from build123d import *

# Parameters (mm, degrees)
BOSS_EXTRUDE1_DEPTH = 124.46
BOSS_EXTRUDE2_START = 127
BOSS_EXTRUDE2_DEPTH = 2.54
BOSS_EXTRUDE3_START = -124.46
BOSS_EXTRUDE3_DEPTH = 2.54
CUT_EXTRUDE1_START  = 19.05
SKETCH4_R           = 6.35
CUT_EXTRUDE1_DEPTH  = 2.54
FILLET1_R           = 2.54
FILLET2_R           = 2.54


with BuildPart() as part:
    # Sketch1 → Boss-Extrude1 (new, symmetric)
    with BuildSketch(Plane(origin=(0, 0, 0), x_dir=(0, 0, -1), z_dir=(1, 0, 0))):
        with BuildLine():
            Line((-16.51, 38.1), (-19.05, 38.1))
            Line((-19.05, 38.1), (-19.05, 2.54))
            ThreePointArc((-19.05, 2.54), (-18.306051224, 0.743948776), (-16.51, 0))
            Line((-16.51, 0), (0, 0))
            Line((0, 0), (0, 1.016))
            Line((0, 1.016), (-6.35, 1.016))
            Line((-6.35, 1.016), (-6.35, 2.54))
            Line((-6.35, 2.54), (-16.51, 2.54))
            Line((-16.51, 2.54), (-16.51, 38.1))
        make_face()
        with BuildLine():
            Line((0, 1.016), (0, 0))
            Line((0, 0), (16.51, 0))
            ThreePointArc((16.51, 0), (18.306051224, 0.743948776), (19.05, 2.54))
            Line((19.05, 2.54), (19.05, 38.1))
            Line((19.05, 38.1), (16.51, 38.1))
            Line((16.51, 38.1), (16.51, 2.54))
            Line((16.51, 2.54), (6.35, 2.54))
            Line((6.35, 2.54), (6.35, 1.016))
            Line((6.35, 1.016), (0, 1.016))
        make_face()
    extrude(amount=BOSS_EXTRUDE1_DEPTH, both=True)

    # Sketch3 → Boss-Extrude2 (add)
    with BuildSketch(Plane(origin=(0, 0, 0), x_dir=(0, 0, -1), z_dir=(1, 0, 0)).offset(BOSS_EXTRUDE2_START)):
        with BuildLine():
            Line((0, 38.1), (-19.05, 38.1))
            Line((-19.05, 38.1), (-19.05, 2.54))
            ThreePointArc((-19.05, 2.54), (-18.306051224, 0.743948776), (-16.51, 0))
            Line((-16.51, 0), (0, 0))
            Line((0, 0), (0, 38.1))
        make_face()
        with BuildLine():
            Line((19.05, 38.1), (0, 38.1))
            Line((0, 38.1), (0, 0))
            Line((0, 0), (16.51, 0))
            ThreePointArc((16.51, 0), (18.306051224, 0.743948776), (19.05, 2.54))
            Line((19.05, 2.54), (19.05, 38.1))
        make_face()
    extrude(amount=-BOSS_EXTRUDE2_DEPTH)

    # Sketch3<4> → Boss-Extrude3 (add)
    with BuildSketch(Plane(origin=(0, 0, 0), x_dir=(0, 0, -1), z_dir=(1, 0, 0)).offset(BOSS_EXTRUDE3_START)):
        with BuildLine():
            Line((0, 38.1), (-19.05, 38.1))
            Line((-19.05, 38.1), (-19.05, 2.54))
            ThreePointArc((-19.05, 2.54), (-18.306051224, 0.743948776), (-16.51, 0))
            Line((-16.51, 0), (0, 0))
            Line((0, 0), (0, 38.1))
        make_face()
        with BuildLine():
            Line((19.05, 38.1), (0, 38.1))
            Line((0, 38.1), (0, 0))
            Line((0, 0), (16.51, 0))
            ThreePointArc((16.51, 0), (18.306051224, 0.743948776), (19.05, 2.54))
            Line((19.05, 2.54), (19.05, 38.1))
        make_face()
    extrude(amount=-BOSS_EXTRUDE3_DEPTH)

    # Sketch4 → Cut-Extrude1 (cut)
    with BuildSketch(Plane.XY.offset(CUT_EXTRUDE1_START)):
        with Locations((-116.84, 10.16)):
            Circle(SKETCH4_R)
    extrude(amount=-CUT_EXTRUDE1_DEPTH, mode=Mode.SUBTRACT)

    # Fillet1
    fillet1_edges = [part.edges().sort_by_distance(p)[0] for p in [
        (-127, 0.743948776, -18.306051224),
        (-127, 0, 0),
        (-127, 0.743948776, 18.306051224),
        (-127, 20.32, 19.05),
        (-127, 20.32, -19.05),
    ]]
    fillet(fillet1_edges, radius=FILLET1_R)

    # Fillet2
    fillet2_edges = [part.edges().sort_by_distance(p)[0] for p in [
        (127, 0, 0),
        (127, 20.32, 19.05),
        (127, 0.743948776, -18.306051224),
        (127, 20.32, -19.05),
        (127, 0.743948776, 18.306051224),
    ]]
    fillet(fillet2_edges, radius=FILLET2_R)


solid = part.part
Verification items for the finished model (mm, model axes). A direction names the side the tool comes from. Round coordinates to 2 decimals unless told otherwise and drop trailing zeros. Order: outer loops, then holes, each group sorted by start corner. A loop starts at its lowest first (then second) coordinate and runs counter-clockwise, first axis right, second up. Notation, with made-up numbers: (36, -25) -> (67, -25) arc R22 cw to (67, 5) -> close; hole circle Ø11 at (11.5, 42). An arc over 180 degrees is marked (long way). Put each result on its own line as item: value.
1) Section check B-B (x = -116.84). Record the cut outline in (y, z).
Final values:
outline: (0, -16.51) arc R2.54 ccw to (2.54, -19.05) -> (38.1, -19.05) -> (38.1, -16.51) -> (2.54, -16.51) -> (2.54, -6.35) -> (1.02, -6.35) -> (1.02, 6.35) -> (2.54, 6.35) -> (2.54, 16.51) -> (3.81, 16.51) -> (3.81, 19.05) -> (2.54, 19.05) arc R2.54 ccw to (0, 16.51) -> close; (16.51, 16.51) -> (38.1, 16.51) -> (38.1, 19.05) -> (16.51, 19.05) -> close
2) Section check A-A (y = 20). Record the cut outline in (x, z), then the cut area to 3 significant figures.
Final values:
outline: (-127, -16.51) arc R2.54 ccw to (-124.46, -19.05) -> (124.46, -19.05) arc R2.54 ccw to (127, -16.51) -> (127, 16.51) arc R2.54 ccw to (124.46, 19.05) -> (-124.46, 19.05) arc R2.54 ccw to (-127, 16.51) -> close; hole (-124.46, -16.51) -> (124.46, -16.51) -> (124.46, 16.51) -> (-124.46, 16.51) -> close
area: 1,450 mm^2
3) Section check D-D (z = 2.5). Record the cut outline in (x, y).
Final values:
outline: (-127, 2.54) arc R2.54 ccw to (-124.46, 0) -> (124.46, 0) arc R2.54 ccw to (127, 2.54) -> (127, 38.1) -> (124.46, 38.1) -> (124.46, 1.02) -> (-124.46, 1.02) -> (-124.46, 38.1) -> (-127, 38.1) -> close
4) Material ranges on line 1 (X direction, y = 27, z = -13.5); line 2 (X direction, y = 10, z = 17); line 3 (Z direction, x = 76, y = 8), recorded low to high.
Final values:
line 1: x = -127 to -124.46, 124.46 to 127
line 2: x = -126.95 to -123.19, -110.49 to 126.95
line 3: z = -19.05 to -16.51, 16.51 to 19.05
5) Depth check by flat-ended pin: pin 1 (5 mm diameter, centred on x = 42, z = 11, fed in from +Y); pin 2 (0.5 mm diameter, centred on x = 15, y = 1.5, fed in from -Z); pin 3 (6.5 mm diameter, centred on x = 8.5, z = 2, fed in from +Y). Enter the tip coordinate at first touch or a pass-through.
Final values:
pin 1: stops at y = 2.54
pin 2: stops at z = -18.92
pin 3: stops at y = 1.02
6) Set-up check for faces 4 (the flat face through (1, 38.1, -17)), 5 (the cylindrical face through (-118.22, 3.96, 17.8)), 6 (the flat face through (2, 1.016, 0)): record each of +Z, -Z, +X, -X, +Y, -Y from which the full face is reachable in a straight line by a thin tool's end or side.
Final values:
face 4: +Z, -Z, +X, -X, +Y
face 5: +Z
face 6: +Y
7) Mould release check, pull along Z, two halves, no side actions. Record for faces 1 (the flat face through (124.46, 20, 0)), 2 (the flat face through (2, 0, 0)), 3 (the flat face through (2, 20, -19.05)): +Z half, -Z half, draft (parallel to the pull), parting line (faces both ways), or undercut.
Final values:
face 1: undercut
face 2: draft
face 3: -Z half
8) Section check C-C (x = 82.5). Record the cut outline in (y, z).
Final values:
outline: (0, -16.51) arc R2.54 ccw to (2.54, -19.05) -> (38.1, -19.05) -> (38.1, -16.51) -> (2.54, -16.51) -> (2.54, -6.35) -> (1.02, -6.35) -> (1.02, 6.35) -> (2.54, 6.35) -> (2.54, 16.51) -> (38.1, 16.51) -> (38.1, 19.05) -> (2.54, 19.05) arc R2.54 ccw to (0, 16.51) -> close
